```python
from build123d import *

# Parameters (mm, degrees)
F1_DEPTH  = 50.8
F2_W      = 6.35
F2_H      = 6.35
F3_DEPTH  = 50.8
F4_W      = 6.35
F4_H      = 6.35
F5_DEPTH  = 50.8
F6_W      = 6.35
F6_H      = 6.35
F7_DEPTH  = 34.925
F9_W      = 101.6
F9_H      = 63.5
F10_DEPTH = 6.35


with BuildPart() as f1:
    # F0 (on Front) → F1 (new body)
    with BuildSketch(Plane.XZ):
        Polygon((-41.275, -3.175), (-34.925, -3.175), (-34.925, 0), (-34.925, 3.175), (-41.275, 3.175), align=None)
    extrude(amount=F1_DEPTH)

    # F2 (on face) → F3 (join)
    with BuildSketch(Plane.XY.offset(3.175)):
        with Locations((-38.1, -3.175)):
            Rectangle(F2_W, F2_H)
        with Locations((-38.1, -47.625)):
            Rectangle(F2_W, F2_H)
    extrude(amount=F3_DEPTH)

    # F4 (on face) → F5 (join)
    with BuildSketch(Plane.XZ.offset(50.8)):
        with Locations((-38.1, 57.15)):
            Rectangle(F4_W, F4_H)
    extrude(amount=-F5_DEPTH)

    # F6 (on face) → F7 (join)
    with BuildSketch(Plane.YZ.offset(-34.925)):
        with Locations((-47.625, 57.15)):
            Rectangle(F6_W, F6_H)
        with Locations((-3.175, 57.15)):
            Rectangle(F6_W, F6_H)
        with Locations((-47.625, 0)):
            Rectangle(F6_W, F6_H)
    extrude(amount=F7_DEPTH)

    # F8: F1 across plane


with BuildPart() as f1_1:
    add(f1.part)
    add(f1.part.mirror(Plane.YZ))

    # F9 (on face) → F10 (join)
    with BuildSketch(Plane.XY.offset(60.325)):
        with Locations((0, -25.4)):
            Rectangle(F9_W, F9_H)
    extrude(amount=F10_DEPTH)


solid = f1_1.part
```
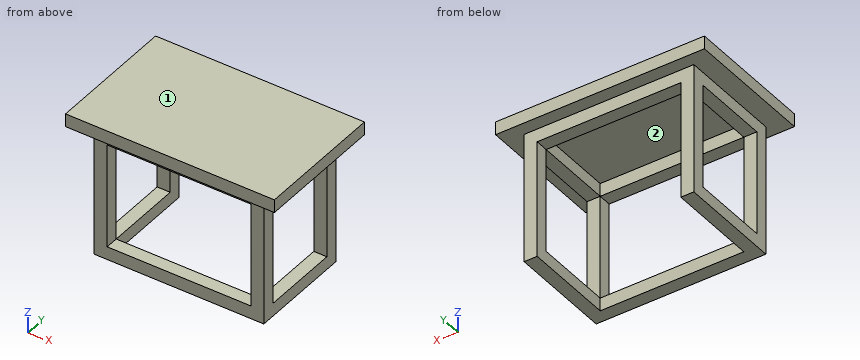
Design review of the part built by this model. Coordinates are the model's own, in mm. Face numbers are marked on the shaded views. Round coordinates to 2 decimals unless told otherwise and drop trailing zeros. Write each loop counter-clockwise with the first axis right and the second up, starting at its lowest first coordinate (ties: lowest second). Pieces come first, ordered by that corner, then holes.
Item 1: We need section C-C on x = 29.5. Write out the cut boundary in (y, z) (3 decimals), and give its area (3 significant figures).
Item 2: The part is to be moulded in two halves that separate along Y. For the marked faces 1 and 2, say which applies: +Y half, -Y half, draft (parallel to the pull), parting line (faces both ways), or undercut.
Item 3: For probe 1 along X at (y, z) = (-45, 28) (3 decimals); probe 2 along Y at (x, z) = (-37, 45); probe 3 along Z at (x, y) = (24, -47) (3 decimals), list the stretches that pass through material, from the lowest coordinate up.
Item 4: We need section D-D on z = 57. Write out the cut boundary in (x, y) (3 decimals), and give its area (3 significant figures).
Item 5: We need section B-B on z = 10. Write out the cut boundary in (x, y) (3 decimals), and give its area (3 significant figures).
Item 6: We need section A-A on y = -15.5. Write out the cut boundary in (x, z) (3 decimals), and give its area (3 significant figures).
Item 7: Clearance check with flat-ended pins moving along their axes: pin 1 Ø3 at (y, z) = (-47, 22.5) entering from +X (3 decimals); pin 2 Ø5 at (x, z) = (-36.5, 36.5) entering from -Y; pin 3 Ø2 at (x, y) = (-20, -34) entering from -Z (3 decimals). State where each tip first meets the part, or that it passes through.
Returned:
1. outline: (-57.15, 60.325) - (-50.8, 60.325) - (-50.8, 53.975) - (-44.45, 53.975) - (-44.45, 60.325) - (-6.35, 60.325) - (-6.35, 53.975) - (0, 53.975) - (0, 60.325) - (6.35, 60.325) - (6.35, 66.675) - (-57.15, 66.675) - close; (-50.8, -3.175) - (-44.45, -3.175) - (-44.45, 3.175) - (-50.8, 3.175) - close
1. area: 524 mm2
2. face 1: draft
2. face 2: undercut
3. probe 1: x = -41.275 to -34.925, 34.925 to 41.275
3. probe 2: y = -50.8 to -44.45, -6.35 to 0
3. probe 3: z = -3.175 to 3.175, 53.975 to 66.675
4. outline: (-41.275, -50.8) - (41.275, -50.8) - (41.275, 0) - (-41.275, 0) - close; hole (-34.925, -44.45) - (34.925, -44.45) - (34.925, -6.35) - (-34.925, -6.35) - close
4. area: 1,530 mm2
5. outline: (-41.275, -50.8) - (-34.925, -50.8) - (-34.925, -44.45) - (-41.275, -44.45) - close; (-41.275, -6.35) - (-34.925, -6.35) - (-34.925, 0) - (-41.275, 0) - close; (34.925, -50.8) - (41.275, -50.8) - (41.275, -44.45) - (34.925, -44.45) - close; (34.925, -6.35) - (41.275, -6.35) - (41.275, 0) - (34.925, 0) - close
5. area: 161 mm2
6. outline: (-50.8, 60.325) - (-41.275, 60.325) - (-41.275, 53.975) - (-34.925, 53.975) - (-34.925, 60.325) - (34.925, 60.325) - (34.925, 53.975) - (41.275, 53.975) - (41.275, 60.325) - (50.8, 60.325) - (50.8, 66.675) - (-50.8, 66.675) - close; (-41.275, -3.175) - (-34.925, -3.175) - (-34.925, 3.175) - (-41.275, 3.175) - close; (34.925, -3.175) - (41.275, -3.175) - (41.275, 3.175) - (34.925, 3.175) - close
6. area: 806 mm2
7. pin 1: stops at x = 41.275
7. pin 2: stops at y = -50.8
7. pin 3: stops at z = 60.325
